Autodesk Inventor part; units mm, degrees
ref_plane "작업 평면1" through (0, 3.4, 0) normal (0, -1, 0) x (1, 0, 0)
ref_plane "YZ Plane" through (0, 0, 0) normal (1, 0, 0) x (0, 1, 0)
ref_plane "XZ Plane" through (0, 0, 0) normal (0, 1, 0) x (-1, 0, 0)
sketch "스케치1" plane through (0, 0, 0) normal (0, 1, 0) x (-1, 0, 0)
  line L0 (-49.8892, 49.8892) -> (-18.2607, 68.1499)
  line L1 (-18.2607, 68.1499) -> (18.2607, 68.1499)
  line L2 (18.2607, 68.1499) -> (49.8892, 49.8892)
  line L3 (49.8892, 49.8892) -> (68.1499, 18.2607)
  line L4 (68.1499, 18.2607) -> (68.1499, -18.2607)
  line L5 (68.1499, -18.2607) -> (49.8892, -49.8892)
  line L6 (49.8892, -49.8892) -> (18.2607, -68.1499)
  line L7 (18.2607, -68.1499) -> (-18.2607, -68.1499)
  line L8 (-18.2607, -68.1499) -> (-49.8892, -49.8892)
  line L9 (-49.8892, -49.8892) -> (-68.1499, -18.2607)
  line L10 (-68.1499, -18.2607) -> (-68.1499, 18.2607)
  line L11 (-68.1499, 18.2607) -> (-49.8892, 49.8892)
  line L12 (71.3499, -19.1182) -> (52.2318, -52.2318)
  line L13 (52.2318, -52.2318) -> (19.1182, -71.3499)
  line L14 (19.1182, -71.3499) -> (-19.1182, -71.3499)
  line L15 (-19.1182, -71.3499) -> (-52.2318, -52.2318)
  line L16 (-52.2318, -52.2318) -> (-71.3499, -19.1182)
  line L17 (-71.3499, -19.1182) -> (-71.3499, 19.1182)
  line L18 (-71.3499, 19.1182) -> (-52.2318, 52.2318)
  line L19 (-52.2318, 52.2318) -> (-19.1182, 71.3499)
  line L20 (-19.1182, 71.3499) -> (19.1182, 71.3499)
  line L21 (19.1182, 71.3499) -> (52.2318, 52.2318)
  line L22 (52.2318, 52.2318) -> (71.3499, 19.1182)
  line L23 (71.3499, 19.1182) -> (71.3499, -19.1182)
  point P0 (0, 0)
  point P1 (0, 0)
  point P2 (0, 0)
  dimension "d0" = 141.108
  dimension "d1" = 3.2
extrude "돌출1" add sketch "스케치1" along normal blind 6.8 contours L0 L1 L2 L3 L4 L5 L6 L7 L8 L9 L10 L11 | L12 L13 L14 L15 L16 L17 L18 L19 L20 L21 L22 L23
sketch "스케치2" plane through (0, 6.8, 0) normal (0, 1, 0) x (1, 0, 0)
  line L0 (-18.6894, 69.7499) -> (18.6894, 69.7499)
  line L1 (18.6894, 69.7499) -> (51.0605, 51.0605)
  line L2 (51.0605, 51.0605) -> (69.7499, 18.6894)
  line L3 (69.7499, 18.6894) -> (69.7499, -18.6894)
  line L4 (69.7499, -18.6894) -> (51.0605, -51.0605)
  line L5 (51.0605, -51.0605) -> (18.6894, -69.7499)
  line L6 (18.6894, -69.7499) -> (-18.6894, -69.7499)
  line L7 (-18.6894, -69.7499) -> (-51.0605, -51.0605)
  line L8 (-51.0605, -51.0605) -> (-69.7499, -18.6894)
  line L9 (-69.7499, -18.6894) -> (-69.7499, 18.6894)
  line L10 (-69.7499, 18.6894) -> (-51.0605, 51.0605)
  line L11 (-51.0605, 51.0605) -> (-18.6894, 69.7499)
  line L12 (-71.3499, 19.1182) -> (-71.3499, -19.1182)
  line L13 (18.1535, -67.7499) -> (-18.1535, -67.7499)
  line L14 (-18.1535, -67.7499) -> (-49.5964, -49.5964)
  line L15 (-49.5964, -49.5964) -> (-67.7499, -18.1535)
  line L16 (-67.7499, -18.1535) -> (-67.7499, 18.1535)
  line L17 (-67.7499, 18.1535) -> (-49.5964, 49.5964)
  line L18 (-49.5964, 49.5964) -> (-18.1535, 67.7499)
  line L19 (-18.1535, 67.7499) -> (18.1535, 67.7499)
  line L20 (18.1535, 67.7499) -> (49.5964, 49.5964)
  line L21 (49.5964, 49.5964) -> (67.7499, 18.1535)
  line L22 (67.7499, 18.1535) -> (67.7499, -18.1535)
  line L23 (67.7499, -18.1535) -> (49.5964, -49.5964)
  line L24 (49.5964, -49.5964) -> (18.1535, -67.7499)
  point P0 (0, 0)
  point P1 (0, 0)
  point P2 (0, 0)
  dimension "d4" = 1.6
  dimension "d5" = 2
extrude "돌출2" cut sketch "스케치2" against normal blind 1.2
sketch "스케치5" plane through (0, 6.8, 0) normal (0, 1, 0) x (1, 0, 0)
  line L0 (-49.5964, -49.5964) -> (-18.1535, -67.7499)
  line L1 (-18.1535, -67.7499) -> (18.1535, -67.7499)
  line L2 (18.1535, -67.7499) -> (49.5964, -49.5964)
  line L3 (49.5964, -49.5964) -> (67.7499, -18.1535)
  line L4 (67.7499, -18.1535) -> (67.7499, 18.1535)
  line L5 (67.7499, 18.1535) -> (49.5964, 49.5964)
  line L6 (49.5964, 49.5964) -> (18.1535, 67.7499)
  line L7 (18.1535, 67.7499) -> (-18.1535, 67.7499)
  line L8 (-18.1535, 67.7499) -> (-49.5964, 49.5964)
  line L9 (-49.5964, 49.5964) -> (-67.7499, 18.1535)
  line L10 (-67.7499, 18.1535) -> (-67.7499, -18.1535)
  line L11 (-67.7499, -18.1535) -> (-49.5964, -49.5964)
  point P0 (0, 0)
extrude "돌출5" cut sketch "스케치5" against normal blind 0.6
fillet "모깎기1" radius 1.2 24 edges at (61.7909, 0, 35.675) (61.7909, 6.8, 35.675) (71.3499, 6.8, 0) (71.3499, 0, 0) (61.7909, 6.8, -35.675) (61.7909, 0, -35.675) (35.675, 6.8, -61.7909) (35.675, 0, -61.7909) (0, 0, -71.3499) (0, 6.8, -71.3499) (-35.675, 6.8, -61.7909) (-35.675, 0, -61.7909) (-61.7909, 0, -35.675) (-61.7909, 6.8, -35.675) (-71.3499, 0, 0) (-71.3499, 6.8, 0) (-61.7909, 0, 35.675) (-61.7909, 6.8, 35.675) (-35.675, 0, 61.7909) (-35.675, 6.8, 61.7909) (0, 0, 71.3499) (0, 6.8, 71.3499) (35.675, 0, 61.7909) (35.675, 6.8, 61.7909)
ref_plane "작업 평면1" through (0, 3.4, 0) normal (0, -1, 0) x (1, 0, 0)
mirror "미러1" about plane through (0, 3.4, 0) normal (0, -1, 0) of "돌출5", "돌출2"
sketch "스케치9" plane through (0, 6.2, 0) normal (0, 1, 0) x (1, 0, 0)
  line L0 (-17.832, -66.5499) -> (-48.7179, -48.7179)
  line L1 (-48.7179, -48.7179) -> (-66.5499, -17.832)
  line L2 (-66.5499, -17.832) -> (-66.5499, 17.832)
  line L3 (-66.5499, 17.832) -> (-48.7179, 48.7179)
  line L4 (-48.7179, 48.7179) -> (-17.832, 66.5499)
  line L5 (-17.832, 66.5499) -> (17.832, 66.5499)
  line L6 (17.832, 66.5499) -> (48.7179, 48.7179)
  line L7 (48.7179, 48.7179) -> (66.5499, 17.832)
  line L8 (66.5499, 17.832) -> (66.5499, -17.832)
  line L9 (66.5499, -17.832) -> (48.7179, -48.7179)
  line L10 (48.7179, -48.7179) -> (17.832, -66.5499)
  line L11 (17.832, -66.5499) -> (-17.832, -66.5499)
  line L12 (18.1535, -67.7499) -> (-18.1535, -67.7499)
  point P0 (0, 0)
  point P1 (0, 0)
  dimension "d37" = 1.2
extrude "돌출9" cut sketch "스케치9" against normal blind 10
properties part number "(x2)_POSPA_Large_Bottom"
Geometry check sheet. Reference: the model listing, model coordinates, mm. A direction names the side the tool comes from. Coordinates: 2 decimals unless noted, no trailing zeros. Order: outer loops, then holes, each group sorted by start corner. A loop starts at its lowest first (then second) coordinate and runs counter-clockwise, first axis right, second up. Notation, with made-up numbers: M 42.5,50 L 58.5,50 A30 ccw 58.5,76 Z; hole C -4.5,-19 d3. An arc over 180 degrees is marked long. Answer as a JSON object with one key per item and string values.
Q1. Cross-section at A-A on x = 6.5. Record the cut outline in (y, z).
Results are:
{"outline": "M 0,-70.15 A1.2 ccw 1.2,-71.35 L 5.6,-71.35 A1.2 ccw 6.8,-70.15 L 6.8,-69.75 L 5.6,-69.75 L 5.6,-67.75 L 6.2,-67.75 L 6.2,-66.55 L 0.6,-66.55 L 0.6,-67.75 L 1.2,-67.75 L 1.2,-69.75 L 0,-69.75 Z; M 0,69.75 L 1.2,69.75 L 1.2,67.75 L 0.6,67.75 L 0.6,66.55 L 6.2,66.55 L 6.2,67.75 L 5.6,67.75 L 5.6,69.75 L 6.8,69.75 L 6.8,70.15 A1.2 ccw 5.6,71.35 L 1.2,71.35 A1.2 ccw 0,70.15 Z"}
Q2. Depth check by flat-ended pin: pin 1 Ø12 at (x, z) = (50, -52) entering from -Y; pin 2 Ø1 at (y, z) = (0.5, -3.5) entering from +X; pin 3 Ø1 at (y, z) = (0.5, -2.5) entering from -X. Enter the tip coordinate at first touch or a pass-through.
Results are:
{"pin 1": "stops at y = 0", "pin 2": "stops at x = 71.33", "pin 3": "stops at x = -71.33"}
Q3. Release check for a two-part mould opening along X. For faces 1 (the flat face through (-30.4, 6.2, -60.5)), 2 (the cylindrical face through (-35.73, 0.34, 61.34)), 3 (the flat face through (35.907, 3.369, 61.657)) record: released by +X, released by -X, zero draft, split by the parting line, or undercut.
Results are:
{"face 1": "undercut", "face 2": "released by -X", "face 3": "released by +X"}
Q4. Tool access check on faces 4 (the flat face through (35.102, 6.208, 60.274)), 5 (the flat face through (66.55, 3, 0)), 6 (the flat face through (33.655, 0.896, 58.8)), 7 (the cylindrical face through (61.36, 6.44, 35.74)), 8 (the flat face through (-71.35, 3, 0)). Record the directions out of +Z, -Z, +X, -X, +Y, -Y that give a thin tool (end or side, any length) a straight path to the whole face; none if there is none.
Results are:
{"face 4": "+Y", "face 5": "+Y, -Y", "face 6": "-Y", "face 7": "+Z, +X, +Y", "face 8": "+Z, -Z, -X, +Y, -Y"}
Q5. Scan lines: line 1 (Z direction, x = 63.5, y = 0.75); line 2 (X direction, y = 3.5, z = 2); line 3 (X direction, y = 2.75, z = 36). Record each from-to range of solid material in increasing order.
Results are:
{"line 1": "z = -32.54 to -29.51, -25.51 to -23.11, 23.11 to 25.51, 29.51 to 32.54", "line 2": "x = -71.35 to -66.55, 66.55 to 71.35", "line 3": "x = -61.6 to -56.06, 56.06 to 61.6"}
Q6. Cross-section at B-B on y = 4. Record the cut outline in (x, z), and give its area (3 significant figures).
Results are:
{"outline": "M -71.35,-19.12 L -52.23,-52.23 L -19.12,-71.35 L 19.12,-71.35 L 52.23,-52.23 L 71.35,-19.12 L 71.35,19.12 L 52.23,52.23 L 19.12,71.35 L -19.12,71.35 L -52.23,52.23 L -71.35,19.12 Z; hole M -66.55,-17.83 L -48.72,-48.72 L -17.83,-66.55 L 17.83,-66.55 L 48.72,-48.72 L 66.55,-17.83 L 66.55,17.83 L 48.72,48.72 L 17.83,66.55 L -17.83,66.55 L -48.72,48.72 L -66.55,17.83 Z", "area": "2,130 mm²"}
Q7. Cross-section at C-C on z = -4.5. Record the cut outline in (x, y), and give its area (3 significant figures).
Results are:
{"outline": "M -71.35,1.2 A1.2 ccw -70.15,0 L -69.75,0 L -69.75,1.2 L -67.75,1.2 L -67.75,0.6 L -66.55,0.6 L -66.55,6.2 L -67.75,6.2 L -67.75,5.6 L -69.75,5.6 L -69.75,6.8 L -70.15,6.8 A1.2 ccw -71.35,5.6 Z; M 66.55,0.6 L 67.75,0.6 L 67.75,1.2 L 69.75,1.2 L 69.75,0 L 70.15,0 A1.2 ccw 71.35,1.2 L 71.35,5.6 A1.2 ccw 70.15,6.8 L 69.75,6.8 L 69.75,5.6 L 67.75,5.6 L 67.75,6.2 L 66.55,6.2 Z", "area": "51.6 mm²"}
